Input: dimensioned drawing with shaded views. Units: mm. Origin: part minimum x, y, z. A direction names the side the tool comes from. Round coordinates to 2 decimals unless told otherwise and drop trailing zeros. Loops run counter-clockwise (first coordinate to the right, second up) from the corner with the lowest first, then second, coordinate; pieces in that order, holes last. Notation, with made-up numbers: M 20.5,-24.5 L 24.5,-24.5 A20 cw 24.5,-3.5 Z; hole C 4.5,55 d3. An arc over 180 degrees is marked long. Use one line per item in the form item = value. Start each with the question number.
Q1. Mould query, pull axis X, two halves, no side actions, for the marked faces 1, 2 and 3. Classes: pulls with the +X half, pulls with the -X half, needs draft (parallel to the pull), parting line crosses it, or undercut.
Q2. First-contact query: P1, Ø5, axis at x = 31, y = 10, coming from the +Z side; P2, Ø12, axis at x = 9.5, y = 12.5, coming from the -Z side; P3, Ø4.5, axis at x = 54.5, y = 11.5, coming from the -Z side; P4, Ø10, axis at y = 11.5, z = 11, coming from the +X side. Flat tips, straight axial feed; report the tip coordinate or a pass-through.
Q3. Access query for the marked faces 4, 5 and 6. Directions: +Z, -Z, +X, -X, +Y, -Y. A direction counts if a zero-diameter tool reaches every point of the face in a straight line with its end or side. Return the directions, or none.
Q4. Section query C-C, the plane y = 4. Output: boundary loops of the cut face in (x, z), and give its area (3 significant figures).
Q5. Section query B-B, the plane z = 6.75. Output: boundary loops of the cut face in (x, y), and give its area (3 significant figures).
Q6. Ray query, line 1 along X through (y, z) = (18.5, 9.25); line 2 along Y through (x, z) = (7.5, 25.25); line 3 along X through (y, z) = (15.25, 24). Return the intervals inside material, ascending.
Q7. Section query D-D, the plane y = 11.5. State how many separate pieces and enclosed holes the cut face has, and give its area (3 significant figures).
Q8. Section query A-A, the plane x = 31. Output: boundary loops of the cut face in (y, z).
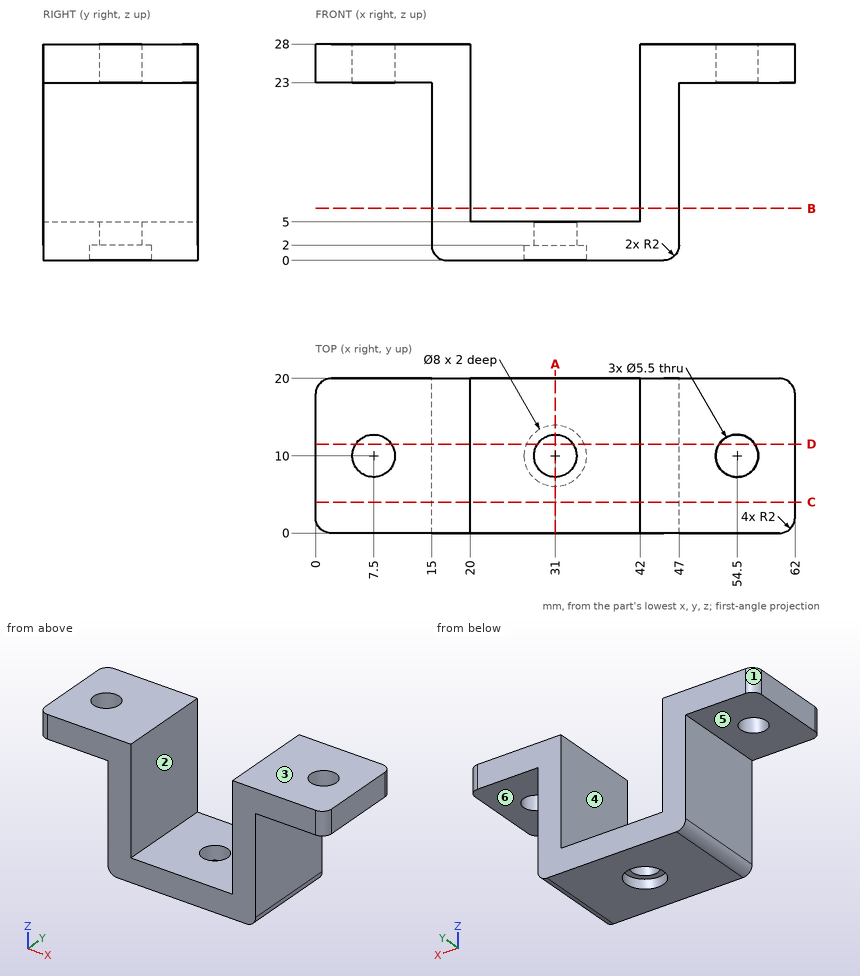
Results found:
q1.face_1 = pulls with the -X half
q1.face_2 = undercut
q1.face_3 = needs draft
q2.P1 = through
q2.P2 = 0.68
q2.P3 = 23
q2.P4 = 47
q3.face_4 = +Z, +Y, -Y
q3.face_5 = -Z, -X, +Y, -Y
q3.face_6 = -Z, +X, +Y, -Y
q4.outline = M 0,23 L 15,23 L 15,2 A2 ccw 17,0 L 45,0 A2 ccw 47,2 L 47,23 L 62,23 L 62,28 L 42,28 L 42,5 L 20,5 L 20,28 L 0,28 Z
q4.area = 538 mm²
q5.outline = M 15,0 L 20,0 L 20,20 L 15,20 Z; M 42,0 L 47,0 L 47,20 L 42,20 Z
q5.area = 200 mm²
q6.line_1 = 15 to 20, 42 to 47
q6.line_2 = 0 to 7.25, 12.75 to 20
q6.line_3 = 0 to 20, 42 to 62
q7.separate_pieces = 4
q7.enclosed_holes = 0
q7.area = 464 mm²
q8.outline = M 0,0 L 6,0 L 6,2 L 7.25,2 L 7.25,5 L 0,5 Z; M 12.75,2 L 14,2 L 14,0 L 20,0 L 20,5 L 12.75,5 Z
